Work out the finished part from the listing and answer in its coordinate system (mm). A direction names the side the tool comes from. Round coordinates to 2 decimals unless told otherwise and drop trailing zeros. Order: outer loops, then holes, each group sorted by start corner. A loop starts at its lowest first (then second) coordinate and runs counter-clockwise, first axis right, second up. Notation, with made-up numbers: (13, 51) - (36, 51) arc R34 cw to (36, 84) - close; hole circle Ø3 at (-27.5, -16.75). An arc over 180 degrees is marked (long way). Answer in a Markdown table with one row per item.
from build123d import *

# Parameters (mm, degrees)
PLATE_DEPTH         = 9
SKETCH3_R           = 1.525
HEX_HOLES_DEPTH     = 128.597021909
SKETCH4_R           = 1.525
ARDUINO_HOLES_DEPTH = 128.597021909
SKETCH5_W           = 45
SKETCH5_H           = 105
CUT_EXTRUDE1_DEPTH  = 128.597021909


with BuildPart() as part:
    # Sketch1 → Plate (new body)
    with BuildSketch(Plane(origin=(0, 0, 0), x_dir=(1, 0, 0), z_dir=(0, 1, 0))):
        with BuildLine():
            Line((-65, -90), (65, -90))
            ThreePointArc((65, -90), (82.67766953, -82.67766953), (90, -65))
            Line((90, -65), (90, 65))
            ThreePointArc((90, 65), (82.67766953, 82.67766953), (65, 90))
            Line((65, 90), (-65, 90))
            ThreePointArc((-65, 90), (-82.67766953, 82.67766953), (-90, 65))
            Line((-90, 65), (-90, -65))
            ThreePointArc((-90, -65), (-82.67766953, -82.67766953), (-65, -90))
        make_face()
    extrude(amount=PLATE_DEPTH)

    # Sketch3 → Hex Holes (cut, through all)
    with BuildSketch(Plane(origin=(0, 9, 0), x_dir=(1, 0, 0), z_dir=(0, 1, 0))):
        with Locations(Location((-65, 80, 0), (0, 0, 270))):
            Circle(SKETCH3_R)
        with Locations(Location((-80, 65, 0), (0, 0, 270))):
            Circle(SKETCH3_R)
        with Locations(Location((80, 65, 0), (0, 0, 270))):
            Circle(SKETCH3_R)
        with Locations(Location((80, -65, 0), (0, 0, 270))):
            Circle(SKETCH3_R)
        with Locations(Location((65, 80, 0), (0, 0, 270))):
            Circle(SKETCH3_R)
        with Locations(Location((65, -80, 0), (0, 0, 270))):
            Circle(SKETCH3_R)
        with Locations(Location((-65, -80, 0), (0, 0, 270))):
            Circle(SKETCH3_R)
        with Locations(Location((-80, -65, 0), (0, 0, 270))):
            Circle(SKETCH3_R)
    extrude(amount=-HEX_HOLES_DEPTH, mode=Mode.SUBTRACT)

    # Sketch4 → Arduino Holes (cut, through all)
    with BuildSketch(Plane(origin=(0, 9, 0), x_dir=(1, 0, 0), z_dir=(0, 1, 0))):
        with Locations(Location((-24.5, -31, 0), (0, 0, 270))):
            Circle(SKETCH4_R)
        with Locations(Location((24.5, -31, 0), (0, 0, 270))):
            Circle(SKETCH4_R)
        with Locations(Location((-19.25, 31, 0), (0, 0, 270))):
            Circle(SKETCH4_R)
        with Locations(Location((19.25, 31, 0), (0, 0, 270))):
            Circle(SKETCH4_R)
    extrude(amount=-ARDUINO_HOLES_DEPTH, mode=Mode.SUBTRACT)

    # Sketch5 → Cut-Extrude1 (cut, through all)
    with BuildSketch(Plane(origin=(0, 9, 0), x_dir=(1, 0, 0), z_dir=(0, 1, 0))):
        with Locations((-67.5, 0)):
            Rectangle(SKETCH5_W, SKETCH5_H)
        with Locations((67.5, 0)):
            Rectangle(SKETCH5_W, SKETCH5_H)
    extrude(amount=-CUT_EXTRUDE1_DEPTH, mode=Mode.SUBTRACT)


solid = part.part
1) The mould has two halves that part along Z. Classify faces 4 (the face through (-1, 4, 90)), 5 (the face through (90, 4, 59)), 6 (the face through (-45, 5, 1)): released by +Z, released by -Z, zero draft, split by the parting line, or undercut.
Filled in:
| item | result |
|---|---|
| face 4 | released by +Z |
| face 5 | zero draft |
| face 6 | undercut |
2) Find section C-C, the plane z = 50. Give the vertices of the cut face in (x, y).
Filled in:
| item | result |
|---|---|
| outline | (-45, 0) - (45, 0) - (45, 9) - (-45, 9) - close |
3) Find section B-B, the plane y = 3.25. Give the number of separate pieces and of enclosed holes in the cut face, then the cut area to 3 significant figures.
Filled in:
| item | result |
|---|---|
| separate pieces | 1 |
| enclosed holes | 12 |
| area | 22,300 mm^2 |
4) Find the intervals of material crossed by probe 1 along X at (y, z) = (2.5, -31) (3 decimals); probe 2 along X at (y, z) = (4, 31) (3 decimals); probe 3 along Z at (x, y) = (-65, 7) (3 decimals), in increasing order. Write a range as from..to.
Filled in:
| item | result |
|---|---|
| probe 1 | x = -45..-20.775, -17.725..17.725, 20.775..45 |
| probe 2 | x = -45..-26.025, -22.975..22.975, 26.025..45 |
| probe 3 | z = -90..-81.525, -78.475..-52.5, 52.5..78.475, 81.525..90 |
5) Which of the six approach directions +Z, -Z, +X, -X, +Y, -Y give full straight-line access (tool end or side, diameter ignored) to faces 1 (the face through (-1, 0, -1)), 2 (the face through (67, 5, 52.5)), 3 (the face through (-68, 5, -52.5))?
Filled in:
| item | result |
|---|---|
| face 1 | +Z, -Z, +X, -X, -Y |
| face 2 | +X, +Y, -Y |
| face 3 | -X, +Y, -Y |
6) Each of these flat-tipped pins is pushed along its axis until it touches: pin 1 (2.5 mm diameter, centred on y = 4.5, z = 11, fed in from +X); pin 2 (1.5 mm diameter, centred on y = 7, z = 46.5, fed in from -X); pin 3 (2.5 mm diameter, centred on x = -68.5, y = 4, fed in from -Z). Where does it stop, or does it pass through?
Filled in:
| item | result |
|---|---|
| pin 1 | stops at x = 45 |
| pin 2 | stops at x = -45 |
| pin 3 | stops at z = -89.9 |
7) Find section A-A, the plane x = -55.5. Give the vertices of the cut face in (y, z).
Filled in:
| item | result |
|---|---|
| outline | (0, -90) - (9, -90) - (9, -52.5) - (0, -52.5) - close; (0, 52.5) - (9, 52.5) - (9, 90) - (0, 90) - close |
